from build123d import *

# Parameters (mm, degrees)
SKETCH_2_R          = 55
EXTRUDE_2_DEPTH     = 22
SKETCH_4_R          = 37.5
SKETCH_4_R_2        = 27
EXTRUDE_3_DEPTH     = 106
CUT_EXTRUDE_1_DEPTH = 132.476233594
SKETCH_6_R          = 27
CUT_EXTRUDE_2_DEPTH = 132.476233594


with BuildPart() as part:
    # 草图2 → 凸台-拉伸2 (new body)
    with BuildSketch(Plane.XY):
        Circle(SKETCH_2_R)
    extrude(amount=EXTRUDE_2_DEPTH)

    # 草图4 → 凸台-拉伸3 (add)
    with BuildSketch(Plane.XY.offset(22)):
        Circle(SKETCH_4_R)
        Circle(SKETCH_4_R_2, mode=Mode.SUBTRACT)
    extrude(amount=EXTRUDE_3_DEPTH)

    # 草图5 → 切除-拉伸1 (cut, through all)
    with BuildSketch(Plane.XY.offset(22)):
        with BuildLine():
            ThreePointArc((-54.856374593, 0), (-47.356374593, -7.5), (-39.856374593, 0))
            Line((-39.856374593, 0), (-54.856374593, 0))
        make_face()
        with BuildLine():
            Line((-54.856374593, 0), (-39.856374593, 0))
            ThreePointArc((-39.856374593, 0), (-47.356374593, 7.5), (-54.856374593, 0))
        make_face()
        with BuildLine():
            ThreePointArc((54.149750432, 0), (46.649750432, 7.5), (39.149750432, 0))
            Line((39.149750432, 0), (54.149750432, 0))
        make_face()
        with BuildLine():
            Line((54.149750432, 0), (39.149750432, 0))
            ThreePointArc((39.149750432, 0), (46.649750432, -7.5), (54.149750432, 0))
        make_face()
    extrude(amount=-CUT_EXTRUDE_1_DEPTH, mode=Mode.SUBTRACT)

    # 草图6 → 切除-拉伸2 (cut, through all)
    with BuildSketch(Plane.XY.offset(22)):
        Circle(SKETCH_6_R)
    extrude(amount=-CUT_EXTRUDE_2_DEPTH, mode=Mode.SUBTRACT)


solid = part.part
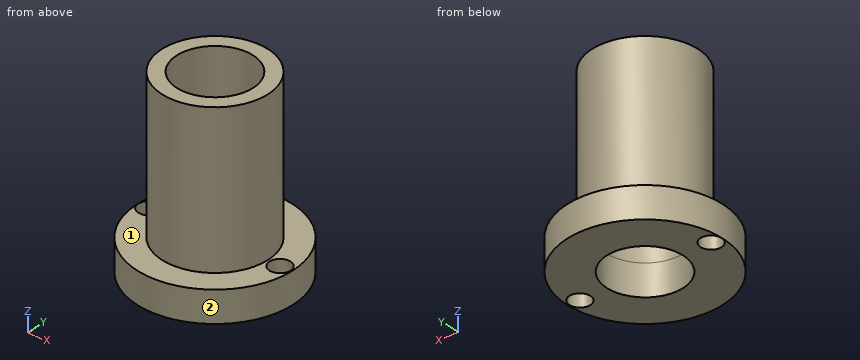
Verification items for the finished model (mm, model axes). Face numbers are marked on the shaded views. A direction names the side the tool comes from. Give positions to 0.01 mm unless a question says otherwise; leave off trailing zeros. Order: outer loops, then holes, each group sorted by start corner. A loop starts at its lowest first (then second) coordinate and runs counter-clockwise, first axis right, second up. Notation, with made-up numbers: M 76,9.5 L 102,9.5 A22 ccw 102,23.5 Z; hole C 7.25,30.25 d10. An arc over 180 degrees is marked long. Use one line per item in the form item = value. Start each with the question number.
Q1. Section check D-D (z = 115). Enter the section's corners in (x, y), then the cut area to 3 significant figures.
Q2. Access from +Z, -Z, +X, -X, +Y, -Y to the whole of each face (thin tool, end or side, straight path). Record for the marked faces 1 and 2.
Q3. Section check C-C (y = -17). Enter the section's corners in (x, z).
Q4. Go/stop test with flat-tipped pins: pin 1 Ø12 at (x, y) = (-47.36, 0) entering from +Z; pin 2 Ø5 at (x, z) = (9.5, 81.5) entering from -Y; pin 3 Ø12 at (y, z) = (-20, 29.5) entering from -X; pin 4 Ø3 at (x, y) = (-37.5, -42) entering from -Z. Record where each tip stops, or that it passes through.
Q5. Scan lines: line 1 along Y through (x, z) = (0, 91); line 2 along Z through (x, y) = (-35, 41); line 3 along Y through (x, z) = (20.5, 10). Record each from-to range of solid material in increasing order. Write a range as [from, to].
Q6. Section check A-A (x = 0). Enter the section's corners in (y, z).
Q7. Section check B-B (y = 0). Enter the section's corners in (x, z), then the cut area to 3 significant figures.
Evaluation:
q1.outline = C 0,0 d75; hole C 0,0 d54
q1.area = 2,130 mm2
q2.face_1 = +Z
q2.face_2 = +Z, -Z
q3.outline = M -52.31,0 L -20.98,0 L -20.98,128 L -33.43,128 L -33.43,22 L -52.31,22 Z; M 20.98,0 L 52.31,0 L 52.31,22 L 33.43,22 L 33.43,128 L 20.98,128 Z
q4.pin_1 = through
q4.pin_2 = -36.84
q4.pin_3 = -34.79
q4.pin_4 = 0
q5.line_1 = [-37.5, -27], [27, 37.5]
q5.line_2 = [0, 22]
q5.line_3 = [-51.04, -17.57], [17.57, 51.04]
q6.outline = M -55,0 L -27,0 L -27,128 L -37.5,128 L -37.5,22 L -55,22 Z; M 27,0 L 55,0 L 55,22 L 37.5,22 L 37.5,128 L 27,128 Z
q7.outline = M -55,0 L -54.86,0 L -54.86,22 L -55,22 Z; M -39.86,0 L -27,0 L -27,128 L -37.5,128 L -37.5,22 L -39.86,22 Z; M 27,0 L 39.15,0 L 39.15,22 L 37.5,22 L 37.5,128 L 27,128 Z; M 54.15,0 L 55,0 L 55,22 L 54.15,22 Z
q7.area = 2,800 mm2
